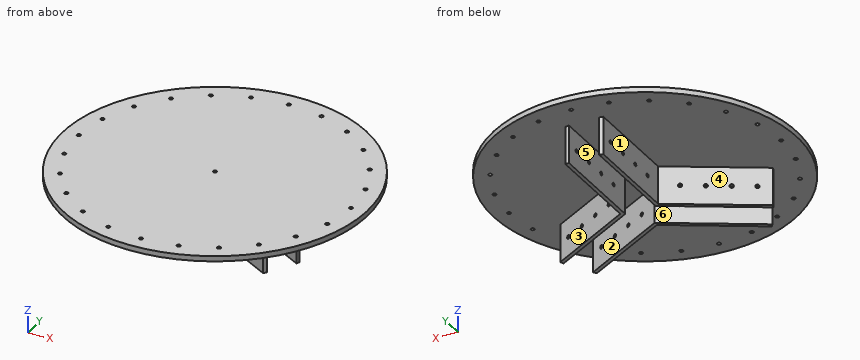
```python
from build123d import *

# Parameters (mm, degrees)
BOSS_EXTRUDE2_DEPTH   = 50
BOSS_EXTRUDE2_2_DEPTH = 50
BOSS_EXTRUDE2_3_DEPTH = 50
SKETCH3_R             = 200
BOSS_EXTRUDE3_DEPTH   = 7
SKETCH4_R             = 2.5
CUT_EXTRUDE1_DEPTH    = 170
CIRPATTERN1_COUNT     = 3
SKETCH5_R             = 2.5
CUT_EXTRUDE2_DEPTH    = 170
CIRPATTERN2_COUNT     = 24


with BuildPart() as part:
    # Sketch2 → Boss-Extrude2 (new body)
    with BuildSketch(Plane.XY):
        with BuildLine():
            Line((0, -23.094010768), (118.743931896, -91.650851812))
            ThreePointArc((118.743931896, -91.650851812), (117.182059436, -93.639547982), (115.586884574, -95.601632383))
            Line((115.586884574, -95.601632383), (0, -28.867513459))
            Line((0, -28.867513459), (-115.586884574, -95.601632383))
            ThreePointArc((-115.586884574, -95.601632383), (-117.182059436, -93.639547982), (-118.743931896, -91.650851812))
            Line((-118.743931896, -91.650851812), (0, -23.094010768))
        make_face()
    extrude(amount=BOSS_EXTRUDE2_DEPTH)



with BuildPart() as body_2:
    # Sketch2 → Boss-Extrude2 2 (new body)
    with BuildSketch(Plane.XY):
        with BuildLine():
            Line((20, 11.547005384), (138.743931896, -57.009835661))
            ThreePointArc((138.743931896, -57.009835661), (139.68525707, -54.662866348), (140.586884574, -52.300362194))
            Line((140.586884574, -52.300362194), (25, 14.43375673))
            Line((25, 14.43375673), (25, 147.901994577))
            ThreePointArc((25, 147.901994577), (22.503197633, 148.302414331), (20, 148.660687473))
            Line((20, 148.660687473), (20, 11.547005384))
        make_face()
    extrude(amount=BOSS_EXTRUDE2_2_DEPTH)


with BuildPart() as body_3:
    # Sketch2 → Boss-Extrude2 3 (new body)
    with BuildSketch(Plane.XY):
        with BuildLine():
            Line((-20, 11.547005384), (-20, 148.660687473))
            ThreePointArc((-20, 148.660687473), (-22.503197633, 148.302414331), (-25, 147.901994577))
            Line((-25, 147.901994577), (-25, 14.43375673))
            Line((-25, 14.43375673), (-140.586884574, -52.300362194))
            ThreePointArc((-140.586884574, -52.300362194), (-139.68525707, -54.662866348), (-138.743931896, -57.009835661))
            Line((-138.743931896, -57.009835661), (-20, 11.547005384))
        make_face()
    extrude(amount=BOSS_EXTRUDE2_3_DEPTH)


with BuildPart() as part_1:
    add(part.part)

    add(body_2.part)  # Boss-Extrude3 merges body 2

    add(body_3.part)  # Boss-Extrude3 merges body 3
    # Sketch3 → Boss-Extrude3 (add)
    with BuildSketch(Plane.XY.offset(50)):
        Circle(SKETCH3_R)
    extrude(amount=BOSS_EXTRUDE3_DEPTH)

    # Sketch4 → Cut-Extrude1 (cut, symmetric)
    with BuildSketch(Plane(origin=(0, 0, 0), x_dir=(0, 0, -1), z_dir=(1, 0, 0))):
        with Locations(Location((-25, 40, 0), (0, 0, 270))):
            Circle(SKETCH4_R)
        with Locations(Location((-25, 70, 0), (0, 0, 270))):
            Circle(SKETCH4_R)
        with Locations(Location((-25, 100, 0), (0, 0, 270))):
            Circle(SKETCH4_R)
        with Locations(Location((-25, 130, 0), (0, 0, 270))):
            Circle(SKETCH4_R)
    cut_extrude1 = extrude(amount=CUT_EXTRUDE1_DEPTH, both=True, mode=Mode.SUBTRACT)

    # CirPattern1: Cut-Extrude1 ×3 about axis
    cirpattern1_axis = Axis((0, 0, 50), (0, 0, 1))
    for i in range(1, CIRPATTERN1_COUNT):
        add(cut_extrude1.rotate(cirpattern1_axis, i * 360 / CIRPATTERN1_COUNT), mode=Mode.SUBTRACT)

    # Sketch5 → Cut-Extrude2 (cut)
    with BuildSketch(Plane.XY.offset(57)):
        Circle(SKETCH5_R)
        with Locations((180, 0)):
            Circle(SKETCH5_R)
    cut_extrude2 = extrude(amount=-CUT_EXTRUDE2_DEPTH, mode=Mode.SUBTRACT)

    # CirPattern2: Cut-Extrude2 ×24 about axis
    cirpattern2_axis = Axis((0, 0, 0), (0, 0, 1))
    for i in range(1, CIRPATTERN2_COUNT):
        add(cut_extrude2.rotate(cirpattern2_axis, i * 360 / CIRPATTERN2_COUNT), mode=Mode.SUBTRACT)


solid = part_1.part
```
Could you check a few things on this model? Use its own coordinates, in mm. Face numbers are marked on the shaded views. A direction names the side the tool comes from. Coordinates: 2 decimals unless noted, no trailing zeros. Write each loop counter-clockwise with the first axis right and the second up, starting at its lowest first coordinate (ties: lowest second). Pieces come first, ordered by that corner, then holes. Notation, with made-up numbers: M -3,32 L 4,32 A19 ccw 4,58 Z; hole C 68.25,10.25 d5. An arc over 180 degrees is marked long. Answer as CSV lines item,"result". Start each with the question number.
1) I want a section at A-A, the plane z = 38. Please give me the cut outline in (x, y), and give its area (3 significant figures).
2) Please list where these lines run through material, in increasing order: line 1 (X direction, y = 129, z = 52.5); line 2 (X direction, y = -90, z = 54); line 3 (Y direction, x = -21.4, z = 25). Write a range as from..to.
3) For P1, Ø6.5, axis at y = 130, z = 25, coming from the -X side; P2, Ø6.5, axis at y = 70, z = 25, coming from the +X side; P3, Ø3, axis at x = 46.59, y = 173.87, coming from the -Z side; P4, Ø6.5, axis at x = 0, y = 180, coming from the -Z side, each with a flat end and sliding along its axis, tell me the tip position at first contact or that it passes through.
4) I want a section at B-B, the plane y = 21. Please give me the cut outline in (x, z), and give its area (3 significant figures).
5) I want a section at C-C, the plane x = 163. Please give me the cut outline in (y, z).
6) I want a section at D-D, the plane y = 166. Please give me the cut outline in (x, z).
7) For the marked faces 4, 5 and 6, which set-ups out of +Z, -Z, +X, -X, +Y, -Y let a thin tool reach every point of the face, with its end or its side?
8) We'd pull the mould along Y, two halves only. Please class the marked faces 1, 2 and 3: +Y half, -Y half, draft (parallel to the pull), parting line (faces both ways), or undercut.
Data:
1,outline,"M -140.59,-52.3 A150 ccw -138.74,-57.01 L -20,11.55 L -20,148.66 A150 ccw -25,147.9 L -25,14.43 Z; M -118.74,-91.65 A150 ccw -115.59,-95.6 L 0,-28.87 L 115.59,-95.6 A150 ccw 118.74,-91.65 L 0,-23.09 Z; M 20,11.55 L 138.74,-57.01 A150 ccw 140.59,-52.3 L 25,14.43 L 25,147.9 A150 ccw 20,148.66 Z"
1,area,"4,060 mm^2"
2,line 1,"x = -152.84..-129.09, -125.47..125.47, 129.09..152.84"
2,line 2,"x = -178.61..-158.38, -153.38..153.38, 158.38..178.61"
2,line 3,"y = -37.93..-35.45, 10.74..37.5, 42.5..67.5, 72.5..97.5, 102.5..127.5, 132.5..148.47"
3,P1,"stops at x = -25"
3,P2,"stops at x = 25"
3,P3,"passes through"
3,P4,"stops at z = 50"
4,outline,"M -198.89,50 L -25,50 L -25,0 L -20,0 L -20,50 L 20,50 L 20,0 L 25,0 L 25,50 L 198.89,50 L 198.89,57 L -198.89,57 Z"
4,area,"3,280 mm^2"
5,outline,"M -115.89,50 L 115.89,50 L 115.89,57 L -115.89,57 Z"
6,outline,"M -111.55,50 L 111.55,50 L 111.55,57 L -111.55,57 Z"
7,face 4,"-Z, -X, +Y"
7,face 5,"-Z, +Y"
7,face 6,"-Z"
8,face 1,"draft"
8,face 2,"undercut"
8,face 3,"+Y half"
